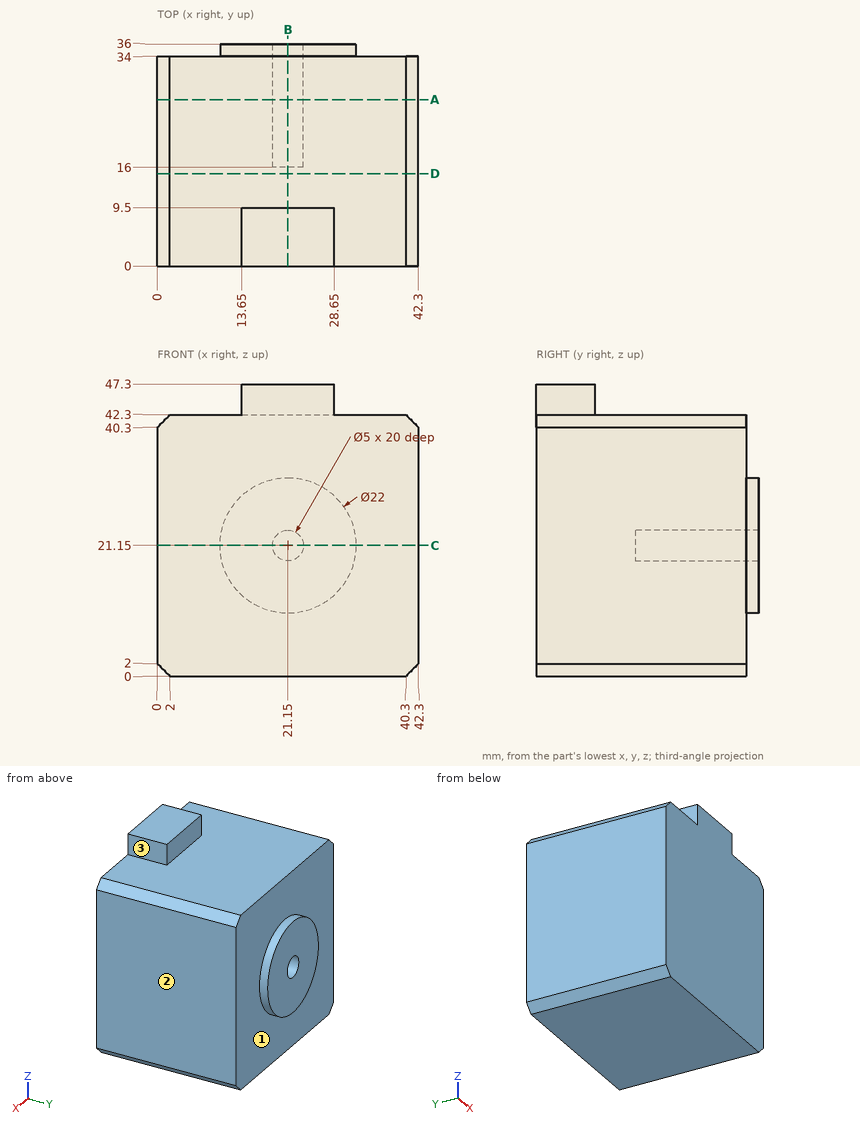
The figure shows three views and two pictorial views of one solid part (mm, origin at its lowest corner). Answer the questions. A direction names the side the tool comes from. Coordinates: 2 decimals unless noted, no trailing zeros. Loops run counter-clockwise (first coordinate to the right, second up) from the corner with the lowest first, then second, coordinate; pieces in that order, holes last. Notation, with made-up numbers: M 9.25,32 L 46.25,32 A24 ccw 46.25,54 Z; hole C 14.25,57 d10. An arc over 180 degrees is marked long. Use CSV: the item, a comma, the result in double quotes. Start each with the question number.
(1) For the marked faces 1, 2 and 3, determine the directions among +Z, -Z, +X, -X, +Y, -Y from which every point of the face is accessible in a straight line to the end or side of a thin tool.
(2) Find section A-A, the plane y = 27. Give the vertices of the cut face in (x, z), then the cut area to 3 significant figures.
(3) Given pin 1 Ø5.5 at (x, z) = (20.5, 21.5) entering from +Y; pin 2 Ø2.5 at (x, z) = (18.5, 45) entering from +Y; pin 3 Ø4 at (y, z) = (4, 45) entering from +X; pin 4 Ø1.5 at (y, z) = (6, 45) entering from -X, each flat-ended and moving along its own axis, determine where each tip first touches the part or whether it passes through.
(4) Find section C-C, the plane z = 21.15. Give the vertices of the cut face in (x, y), then the cut area to 3 significant figures.
(5) Find section B-B, the plane x = 21.15. Give the vertices of the cut face in (y, z), then the cut area to 3 significant figures.
(6) Consider line 1 (X direction, y = 22, z = 21); line 2 (Y direction, x = 35, z = 41.5). Determine where each line is inside the solid, lowest interval first.
(7) Find section D-D, the plane y = 15. Give the vertices of the cut face in (x, z).
Recorded:
1,face 1,"+Y"
1,face 2,"+Z, -Z, +X, +Y, -Y"
1,face 3,"+Z, +X, +Y, -Y"
2,outline,"M 0,2 L 2,0 L 40.3,0 L 42.3,2 L 42.3,40.3 L 40.3,42.3 L 2,42.3 L 0,40.3 Z; hole C 21.15,21.15 d5"
2,area,"1,760 mm^2"
3,pin 1,"stops at y = 36"
3,pin 2,"stops at y = 9.5"
3,pin 3,"stops at x = 28.65"
3,pin 4,"stops at x = 13.65"
4,outline,"M 0,0 L 42.3,0 L 42.3,34 L 32.15,34 L 32.15,36 L 23.65,36 L 23.65,16 L 18.65,16 L 18.65,36 L 10.15,36 L 10.15,34 L 0,34 Z"
4,area,"1,380 mm^2"
5,outline,"M 0,0 L 34,0 L 34,10.15 L 36,10.15 L 36,18.65 L 16,18.65 L 16,23.65 L 36,23.65 L 36,32.15 L 34,32.15 L 34,42.3 L 9.5,42.3 L 9.5,47.3 L 0,47.3 Z"
5,area,"1,430 mm^2"
6,line 1,"x = 0 to 18.65, 23.65 to 42.3"
6,line 2,"y = 0 to 34"
7,outline,"M 0,2 L 2,0 L 40.3,0 L 42.3,2 L 42.3,40.3 L 40.3,42.3 L 2,42.3 L 0,40.3 Z"
